Model file for the job. Use its own axes, mm. A direction names the side the tool comes from. Coordinates: 2 decimals unless noted, no trailing zeros. Write each loop counter-clockwise with the first axis right and the second up, starting at its lowest first coordinate (ties: lowest second). Pieces come first, ordered by that corner, then holes.
Q1. Which spindle directions (+Z, -Z, +X, -X, +Y, -Y) get a long thin tool onto all of the face, cutting with end or side? Do faces 1 (the flat face through (7, 1.588, 0)), 2 (the flat face through (-25.93, 1.93, 0.09)), 3 (the flat face through (-4, 6.35, 0)). Say none if no direction does.
Q2. Band-saw the part on D-D, the plane z = -2.5. Write the cut outline in (x, y).
Q3. Band-saw the part on A-A, the plane x = 0. Write the cut outline in (y, z).
Q4. Pin check, flat tips, straight feed: P1, Ø5, axis at x = 11, z = -3.5, coming from the -Y side; P2, Ø0.7, axis at y = 2.5, z = 0.5, coming from the -X side; P3, Ø4, axis at x = -16.5, z = 3, coming from the -Y side. Stop position of each tip, or through.
Q5. Band-saw the part on C-C, the plane y = 5. Write the cut outline in (x, z) (3 decimals).
Q6. Pull direction Z, two halves, no side cores. Call faces 4 (the cylindrical face through (-28.575, 3.131, 0.09)), 5 (the flat face through (1, 4, 6.35)), 6 (the flat face through (19.05, 4, 0)), 7 (the cylindrical face through (3.05, 3.94, 1.26)): released by +Z, released by -Z, zero draft, split by the parting line, or undercut.
Q7. Drill centre lines: probe 1 along X at (y, z) = (4.9, 0) (3 decimals); probe 2 along Z at (x, y) = (0, 4.9); probe 3 along X at (y, z) = (2.5, 0) (3 decimals). Where is each one in solid material? Low to high.
from build123d import *

# Parameters (mm, degrees)
SKETCH1_R           = 3.302
BOSS_EXTRUDE1_DEPTH = 6.35
CUT_EXTRUDE1_DEPTH  = 13.7


with BuildPart() as part:
    # Sketch1 → Boss-Extrude1 (new body)
    with BuildSketch(Plane(origin=(0, 0, 0), x_dir=(1, 0, 0), z_dir=(0, 1, 0))):
        with BuildLine():
            Line((19.05, 6.35), (19.05, -6.35))
            Line((19.05, -6.35), (-27.86051193, -6.35))
            ThreePointArc((-27.86051193, -6.35), (-28.575, 0), (-27.86051193, 6.35))
            Line((-27.86051193, 6.35), (19.05, 6.35))
        make_face()
        Circle(SKETCH1_R, mode=Mode.SUBTRACT)
    extrude(amount=BOSS_EXTRUDE1_DEPTH)

    # Sketch2 → Cut-Extrude1 (cut, through all)
    with BuildSketch(Plane.XY.offset(6.35)):
        Polygon((19.05, 0), (19.05, 1.5875), (-6.35, 1.5875), (-26.27301193, 1.5875), (-27.86051193, 0), align=None)
        Polygon((-26.27301193, 1.5875), (-6.35, 1.5875), (-6.35, 3.81), (-24.05051193, 3.81), align=None)
    extrude(amount=-CUT_EXTRUDE1_DEPTH, mode=Mode.SUBTRACT)


solid = part.part
Answer sheet:
1. face 1: +Z, -Z, +X, -Y
1. face 2: +Z, -Z, -Y
1. face 3: +Z, -Z, +X, -X, +Y
2. outline: (-28.47, 0) - (-27.86, 0) - (-24.05, 3.81) - (-6.35, 3.81) - (-6.35, 1.59) - (-2.16, 1.59) - (-2.16, 6.35) - (-28.47, 6.35) - close; (2.16, 1.59) - (19.05, 1.59) - (19.05, 6.35) - (2.16, 6.35) - close
3. outline: (1.59, -6.35) - (6.35, -6.35) - (6.35, -3.3) - (1.59, -3.3) - close; (1.59, 3.3) - (6.35, 3.3) - (6.35, 6.35) - (1.59, 6.35) - close
4. P1: stops at y = 1.59
4. P2: stops at x = -28.57
4. P3: stops at y = 3.81
5. outline: (-27.861, -6.35) - (19.05, -6.35) - (19.05, 6.35) - (-27.861, 6.35) arc R28.575 ccw to start; hole circle Ø6.604 at (0, 0)
6. face 4: split by the parting line
6. face 5: released by +Z
6. face 6: zero draft
6. face 7: undercut
7. probe 1: x = -28.575 to -3.302, 3.302 to 19.05
7. probe 2: z = -6.35 to -3.3, 3.3 to 6.35
7. probe 3: x = -28.575 to -25.361, -6.35 to -3.302, 3.302 to 19.05
